Here's how the part is built. I have some questions about the finished solid (model axes, mm). A direction names the side the tool comes from. Give positions to 0.01 mm unless a question says otherwise; leave off trailing zeros. Order: outer loops, then holes, each group sorted by start corner. A loop starts at its lowest first (then second) coordinate and runs counter-clockwise, first axis right, second up.
from build123d import *

# Parameters (mm, degrees)
RESSALTO_EXTRUS_O1_DEPTH = 30.8
ESBO_O2_R                = 1.5
CORTE_EXTRUS_O1_DEPTH    = 30.8


with BuildPart() as part:
    # Esboço1 → Ressalto-extrusão1 (new body)
    with BuildSketch(Plane.XY):
        with BuildLine():
            Line((-8.5, 6.5), (8.5, 6.5))
            Line((8.5, 6.5), (8.5, 0))
            Line((8.5, 0), (3.5, 0))
            Line((3.5, 0), (3.5, 0.8))
            ThreePointArc((3.5, 0.8), (4.3, 1.6), (3.5, 2.4))
            Line((3.5, 2.4), (3.5, 3.2))
            Line((3.5, 3.2), (-3.5, 3.2))
            Line((-3.5, 3.2), (-3.5, 2.4))
            ThreePointArc((-3.5, 2.4), (-4.3, 1.6), (-3.5, 0.8))
            Line((-3.5, 0.8), (-3.5, 0))
            Line((-3.5, 0), (-8.5, 0))
            Line((-8.5, 0), (-8.5, 6.5))
        make_face()
    extrude(amount=RESSALTO_EXTRUS_O1_DEPTH)

    # Esboço2 → Corte-extrusão1 (cut)
    with BuildSketch(Plane(origin=(0, 6.5, 0), x_dir=(1, 0, 0), z_dir=(0, 1, 0))):
        with Locations((6, -21.9)):
            Circle(ESBO_O2_R)
        with Locations((6, -8.9)):
            Circle(ESBO_O2_R)
        with Locations((-6, -21.9)):
            Circle(ESBO_O2_R)
        with Locations((-6, -8.9)):
            Circle(ESBO_O2_R)
    extrude(amount=-CORTE_EXTRUS_O1_DEPTH, mode=Mode.SUBTRACT)


solid = part.part
Q1. If we section it at A-A on y = 4.25: List the corners of the cut face in (x, z) for me.
Filled sheet:
outline: (-8.5, 0) - (8.5, 0) - (8.5, 30.8) - (-8.5, 30.8) - close; hole circle Ø3 at (-6, 8.9); hole circle Ø3 at (-6, 21.9); hole circle Ø3 at (6, 8.9); hole circle Ø3 at (6, 21.9)
Q2. I'm going to push flat-ended pins straight in: P1, Ø4, axis at x = -6, z = 21.9, coming from the -Y side; P2, Ø5.5, axis at x = 0.5, z = 10.5, coming from the -Y side. Where does each tip first touch, or does it pass through?
Filled sheet:
P1: stops at y = 0
P2: stops at y = 3.2
Q3. Thinking about a two-plate mould opening in X: for faces 4 (the face through (8.5, 3, 15)), 5 (the face through (-7.11, 3.3, 20.89)), 6 (the face through (-6, 0, 15)), which applies, released by +X, released by -X, zero draft, split by the parting line, or undercut?
Filled sheet:
face 4: released by +X
face 5: undercut
face 6: zero draft
Q4. If we section it at B-B on x = -6: List the corners of the cut face in (y, z) for me, plus the area to 3 significant figures.
Filled sheet:
outline: (0, 0) - (6.5, 0) - (6.5, 7.4) - (0, 7.4) - close; (0, 10.4) - (6.5, 10.4) - (6.5, 20.4) - (0, 20.4) - close; (0, 23.4) - (6.5, 23.4) - (6.5, 30.8) - (0, 30.8) - close
area: 161 mm2
Q5. If we section it at C-C on z = 29: List the corners of the cut face in (x, y) for me, plus the area to 3 significant figures.
Filled sheet:
outline: (-8.5, 0) - (-3.5, 0) - (-3.5, 0.8) arc R0.8 cw to (-3.5, 2.4) - (-3.5, 3.2) - (3.5, 3.2) - (3.5, 2.4) arc R0.8 cw to (3.5, 0.8) - (3.5, 0) - (8.5, 0) - (8.5, 6.5) - (-8.5, 6.5) - close
area: 86.1 mm2
Q6. I need wall thicknesses on L1, parallel to Z at x = 6, y = 2.25; L2, parallel to X at y = 5.25, z = 21.9; L3, parallel to X at y = 2.5, z = 17. Which ranges of each line are inside material? Lowest first, please.
Filled sheet:
L1: z = 0 to 7.4, 10.4 to 20.4, 23.4 to 30.8
L2: x = -8.5 to -7.5, -4.5 to 4.5, 7.5 to 8.5
L3: x = -8.5 to -3.5, 3.5 to 8.5
Q7. If we section it at D-D on x = -0.5: List the corners of the cut face in (y, z) for me, plus the area to 3 significant figures.
Filled sheet:
outline: (3.2, 0) - (6.5, 0) - (6.5, 30.8) - (3.2, 30.8) - close
area: 102 mm2
Q8. For faces 1 (the face through (3.5, 3, 15)), 2 (the face through (-8.5, 3, 15)), 3 (the face through (4.3, 1.6, 15.2)), which set-ups out of +Z, -Z, +X, -X, +Y, -Y let a thin tool reach every point of the face, with its end or its side?
Filled sheet:
face 1: +Z, -Z, -Y
face 2: +Z, -Z, -X, +Y, -Y
face 3: +Z, -Z
